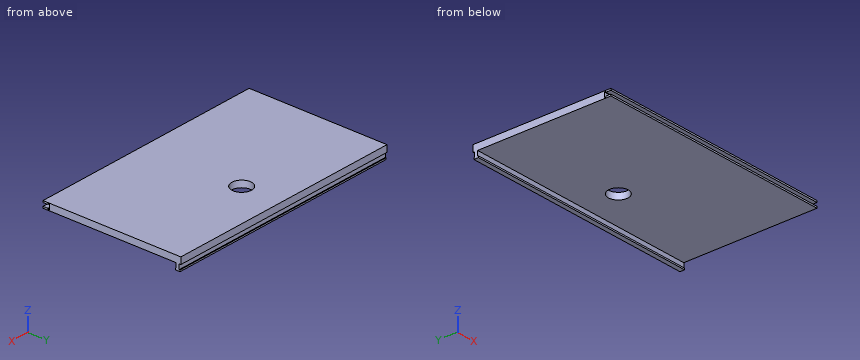
```python
from build123d import *

# Parameters (mm, degrees)
SKETCH150_W     = 145
SKETCH150_H     = 84
SKETCH150_R     = 6
PAD073_DEPTH    = 4
SKETCH179_W     = 1.8
SKETCH179_H     = 3
SKETCH179_W_2   = 2.8
SKETCH179_H_2   = 0.9
PAD084_DEPTH    = 145
SKETCH184_W     = 3
SKETCH184_H     = 2
SKETCH184_W_2   = 1
SKETCH184_H_2   = 3
POCKET108_DEPTH = 145


with BuildPart() as part:
    # Sketch150 → Pad073 (new body)
    with BuildSketch(Plane.XY):
        with Locations((72.5, 42)):
            Rectangle(SKETCH150_W, SKETCH150_H)
        with Locations((74.5, 60)):
            Circle(SKETCH150_R, mode=Mode.SUBTRACT)
    extrude(amount=PAD073_DEPTH)

    # Sketch179 → Pad084 (join)
    with BuildSketch(Plane.YZ):
        with Locations((82.1, -1.5)):
            Rectangle(SKETCH179_W, SKETCH179_H)
        with Locations((82.1, -3.45)):
            Rectangle(SKETCH179_W_2, SKETCH179_H_2)
    extrude(amount=PAD084_DEPTH)

    # Sketch184 → Pocket108 (cut)
    with BuildSketch(Plane.YZ):
        with Locations((1.5, 2)):
            Rectangle(SKETCH184_W, SKETCH184_H)
        with Locations((3.5, 2)):
            Rectangle(SKETCH184_W_2, SKETCH184_H_2)
    extrude(amount=POCKET108_DEPTH, mode=Mode.SUBTRACT)


solid = part.part
```
Can you work these out from the model? Positions are in its coordinate system, mm. Give positions to 0.01 mm unless a question says otherwise; leave off trailing zeros. Loops run counter-clockwise (first coordinate to the right, second up) from the corner with the lowest first, then second, coordinate; pieces in that order, holes last. Notation, with made-up numbers: M -10.5,-18 L 39.5,-18 A7 cw 39.5,-5 Z; hole C -37.5,64 d2. An arc over 180 degrees is marked long. Use one line per item in the form item = value. Start each with the question number.
(1) I want a section at A-A, the plane y = 60. Write out the boundary of the cut face in (x, z), and give its area (3 significant figures).
(2) I want a section at C-C, the plane x = 94. Write out the boundary of the cut face in (y, z), and give its area (3 significant figures).
(3) Please list where these lines run through material, in increasing order: line 1 (Y direction, x = 74.5, z = 3.1); line 2 (Y direction, x = 11, z = 3.25); line 3 (Y direction, x = 74.5, z = 1.4).
(4) I'm going to push flat-ended pins straight in: P1, Ø24.5, axis at x = 67.5, y = 60.5, coming from the -Z side; P2, Ø1.5, axis at x = 80, z = -1, coming from the -Y side; P3, Ø2, axis at x = 50, z = -1.5, coming from the +Y side. Where does each tip first touch, or does it pass through?
(5) I want a section at B-B, the plane x = 74.5. Write out the boundary of the cut face in (y, z), and give its area (3 significant figures).
(6) I want a section at D-D, the plane y = 69. Write out the boundary of the cut face in (x, z).
Worked out:
q1.outline = M 0,0 L 68.5,0 L 68.5,4 L 0,4 Z; M 80.5,0 L 145,0 L 145,4 L 80.5,4 Z
q1.area = 532 mm²
q2.outline = M 0,0 L 81.2,0 L 81.2,-3 L 80.7,-3 L 80.7,-3.9 L 83.5,-3.9 L 83.5,-3 L 83,-3 L 83,0 L 84,0 L 84,4 L 0,4 L 0,3 L 3,3 L 3,3.5 L 4,3.5 L 4,0.5 L 3,0.5 L 3,1 L 0,1 Z
q2.area = 335 mm²
q3.line_1 = 0 to 3, 4 to 54, 66 to 84
q3.line_2 = 0 to 3, 4 to 84
q3.line_3 = 4 to 54, 66 to 84
q4.P1 = 0
q4.P2 = 81.2
q4.P3 = 83
q5.outline = M 0,0 L 54,0 L 54,4 L 0,4 L 0,3 L 3,3 L 3,3.5 L 4,3.5 L 4,0.5 L 3,0.5 L 3,1 L 0,1 Z; M 66,0 L 81.2,0 L 81.2,-3 L 80.7,-3 L 80.7,-3.9 L 83.5,-3.9 L 83.5,-3 L 83,-3 L 83,0 L 84,0 L 84,4 L 66,4 Z
q5.area = 287 mm²
q6.outline = M 0,0 L 145,0 L 145,4 L 0,4 Z
